```python
from build123d import *

# Parameters (mm, degrees)
SKETCH1_R           = 18.5
SKETCH1_R_2         = 6
BOSS_EXTRUDE1_DEPTH = 6
SKETCH2_W           = 5.43768574
SKETCH2_H           = 7.5


with BuildPart() as part:
    # Sketch1 → Boss-Extrude1 (new, symmetric)
    with BuildSketch(Plane(origin=(0, 0, 0), x_dir=(0, 0, -1), z_dir=(1, 0, 0))):
        Circle(SKETCH1_R)
        Circle(SKETCH1_R_2, mode=Mode.SUBTRACT)
    extrude(amount=BOSS_EXTRUDE1_DEPTH, both=True)

    # Sketch2 → Cut-Revolve1 (revolve, cut)
    with BuildSketch(Plane.XY, mode=Mode.PRIVATE) as cut_revolve1_sk:
        with Locations((6, 12.25)):
            Rectangle(SKETCH2_W, SKETCH2_H)
        with Locations((-6, 12.25)):
            Rectangle(SKETCH2_W, SKETCH2_H)
    revolve(cut_revolve1_sk.sketch.rotate(Axis((0, 0, 0), (1, 0, 0)), 90), axis=Axis((0, 0, 0), (1, 0, 0)), mode=Mode.SUBTRACT)


solid = part.part
```
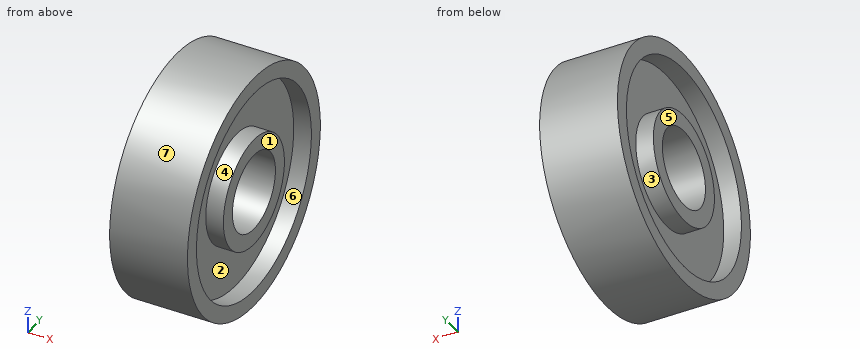
Could you check a few things on this model? Use its own coordinates, in mm. Face numbers are marked on the shaded views. A direction names the side the tool comes from. Round coordinates to 2 decimals unless told otherwise and drop trailing zeros. Write each loop counter-clockwise with the first axis right and the second up, starting at its lowest first coordinate (ties: lowest second). Pieces come first, ordered by that corner, then holes. Notation, with made-up numbers: M -21,-11.5 L 0,-11.5 A28 ccw 0,12.5 Z; hole C 45.5,49.5 d8. An arc over 180 degrees is marked long. Write each question's results on one line, items separated by ' | '. Start each with the question number.
1. I need wall thicknesses on L1, parallel to Y at x = 4.05, z = 0; L2, parallel to Y at x = -4.5, z = -2; L3, parallel to Z at x = -5.25, y = -1.5. Which ranges of each line are inside material? Lowest first, please. Write a range as from..to.
2. Imagine slicing it at D-D on y = 6.5. List the corners of the cut face in (x, z) for me.
3. Imagine slicing it at C-C on x = 4.5. List the corners of the cut face in (y, z) for me, and give its area (3 significant figures).
4. Imagine slicing it at A-A on y = 0. List the corners of the cut face in (x, z) for me.
5. On a 3-axis mill with a long thin cutter (end or side, diameter ignored), from which of +Z, -Z, +X, -X, +Y, -Y can I reach the whole of each face in a straight line? I mean the marked faces 1, 2 and 3. Say none if no direction works.
6. Thinking about a two-plate mould opening in Z: for the marked faces 4, 5, 6 and 7, which applies, +Z half, -Z half, draft (parallel to the pull), parting line (faces both ways), or undercut?
7. I'm going to push flat-ended pins straight in: pin 1 Ø1 at (x, y) = (-4.5, 14.5) entering from +Z; pin 2 Ø3 at (x, y) = (-4.5, 13.5) entering from +Z; pin 3 Ø1.5 at (x, z) = (-0.5, -8.5) entering from +Y; pin 4 Ø16 at (y, z) = (-2.5, 0.5) entering from -X. Where does each tip first touch, or does it pass through?
Result sheet:
1) L1: y = -18.5..-16, -8.5..-6, 6..8.5, 16..18.5 | L2: y = -18.39..-15.87, -8.26..-5.66, 5.66..8.26, 15.87..18.39 | L3: z = -18.44..-15.93, -8.37..-5.81, 5.81..8.37, 15.93..18.44
2) outline: M -6,-17.32 L 6,-17.32 L 6,-14.62 L 3.28,-14.62 L 3.28,-5.48 L 6,-5.48 L 6,5.48 L 3.28,5.48 L 3.28,14.62 L 6,14.62 L 6,17.32 L -6,17.32 L -6,14.62 L -3.28,14.62 L -3.28,5.48 L -6,5.48 L -6,-5.48 L -3.28,-5.48 L -3.28,-14.62 L -6,-14.62 Z
3) outline: C 0,0 d37; C 0,0 d17; hole C 0,0 d32; hole C 0,0 d12 | area: 385 mm^2
4) outline: M -6,-18.5 L 6,-18.5 L 6,-16 L 3.28,-16 L 3.28,-8.5 L 6,-8.5 L 6,-6 L -6,-6 L -6,-8.5 L -3.28,-8.5 L -3.28,-16 L -6,-16 Z; M -6,6 L 6,6 L 6,8.5 L 3.28,8.5 L 3.28,16 L 6,16 L 6,18.5 L -6,18.5 L -6,16 L -3.28,16 L -3.28,8.5 L -6,8.5 Z
5) face 1: +Z, -Z, +X, +Y, -Y | face 2: +X | face 3: -X
6) face 4: undercut | face 5: draft | face 6: undercut | face 7: parting line
7) pin 1: stops at z = 12.09 | pin 2: stops at z = 14.08 | pin 3: stops at y = 16.8 | pin 4: stops at x = -6
